Check sheet for the modelled part. Datum: model origin and axes. Units: mm. A direction names the side the tool comes from. Round coordinates to 2 decimals unless told otherwise and drop trailing zeros. Order: outer loops, then holes, each group sorted by start corner. A loop starts at its lowest first (then second) coordinate and runs counter-clockwise, first axis right, second up. Notation, with made-up numbers: (61, -22.75) -> (93, -22.75) arc R14 cw to (93, -7.75) -> close; hole circle Ø1 at (56.25, 59). An arc over 180 degrees is marked (long way). Answer in a Markdown table with one row per item.
from build123d import *

# Parameters (mm, degrees)
BOSS_EXTRUSION_DEPTH     = 5.5
SCHIZZO2_W               = 14.985516936
SCHIZZO2_H               = 7.7
SCHIZZO2_W_2             = 7.7
SCHIZZO2_H_2             = 15.014483064
SCHIZZO2_W_3             = 15.014483064
SCHIZZO2_H_3             = 15
EXTERNAL_EXTRUSION_DEPTH = 13.5
SCHIZZO3_R               = 2.5
CETRAL_HOLE_DEPTH        = 52.71287379
TAGLIO_ESTRUSIONE2_DEPTH = 57.032066134
TAGLIO_ESTRUSIONE3_DEPTH = 57.021948056
TAGLIO_ESTRUSIONE4_DEPTH = 57.021948056
TAGLIO_ESTRUSIONE5_DEPTH = 57.032066134
FORO_PER_VITE_M4_1_D     = 3
FORO_PER_VITE_M4_2_D     = 3
FORO_PER_VITE_M4_3_D     = 3
FORO_PER_VITE_M4_4_D     = 3
RACCORDO1_R              = 4
RACCORDO2_R              = 4
RACCORDO3_R              = 4
RACCORDO4_R              = 4
RACCORDO5_R              = 2
RACCORDO6_R              = 2
RACCORDO7_R              = 2
RACCORDO8_R              = 2
RACCORDO9_R              = 10
RACCORDO17_R             = 10
RACCORDO18_R             = 10
RACCORDO19_R             = 10
RACCORDO20_R             = 10
RACCORDO21_R             = 10
RACCORDO22_DEPTH         = 5.5
RACCORDO23_R             = 10
RACCORDO24_R             = 10
RACCORDO25_R             = 10


with BuildPart() as part:
    # Schizzo1 → Boss extrusion (new body)
    with BuildSketch(Plane(origin=(0, 0, 0), x_dir=(1, 0, 0), z_dir=(0, 1, 0))):
        Polygon((-3.85, -20.28403897), (-3.85, -35.28403897), (3.85, -35.28403897), (3.85, -20.298522034), (15.500302101, -15.451094793), (20.28403897, -3.85), (35.298522034, -3.85), (35.298522034, 3.85), (20.298522034, 3.85), (15.451094793, 15.500302101), (3.85, 20.28403897), (3.85, 35.298522034), (-3.85, 35.298522034), (-3.85, 20.298522034), (-15.500302101, 15.451094793), (-20.28403897, 3.85), (-35.28403897, 3.85), (-35.28403897, -3.85), (-20.298522034, -3.85), (-15.451094793, -15.500302101), align=None)
    extrude(amount=BOSS_EXTRUSION_DEPTH)

    # Schizzo2 → external extrusion (add)
    with BuildSketch(Plane(origin=(0, 5.5, 0), x_dir=(1, 0, 0), z_dir=(0, 1, 0))):
        with Locations((-27.791280502, 0)):
            Rectangle(SCHIZZO2_W, SCHIZZO2_H)
        with Locations((0, 27.791280502)):
            Rectangle(SCHIZZO2_W_2, SCHIZZO2_H_2)
        with Locations((27.791280502, 0)):
            Rectangle(SCHIZZO2_W_3, SCHIZZO2_H)
        with Locations((0, -27.78403897)):
            Rectangle(SCHIZZO2_W_2, SCHIZZO2_H_3)
    extrude(amount=EXTERNAL_EXTRUSION_DEPTH)

    # Schizzo3 → cetral hole (cut, through all)
    with BuildSketch(Plane(origin=(0, 5.5, 0), x_dir=(1, 0, 0), z_dir=(0, 1, 0))):
        with Locations(Location((0, 0, 0), (0, 0, 270))):
            Circle(SCHIZZO3_R)
    extrude(amount=-CETRAL_HOLE_DEPTH, mode=Mode.SUBTRACT)

    # Schizzo4 → Taglio-Estrusione2 (cut, through all)
    with BuildSketch(Plane.XY.offset(3.85)):
        Polygon((35.298522034, 0), (35.298522034, 19), (31.298522034, 0), align=None)
    extrude(amount=-TAGLIO_ESTRUSIONE2_DEPTH, mode=Mode.SUBTRACT)

    # Schizzo5 → Taglio-Estrusione3 (cut, through all)
    with BuildSketch(Plane(origin=(3.85, 0, 0), x_dir=(0, 0, -1), z_dir=(1, 0, 0))):
        Polygon((35.298522034, 0), (35.298522034, 19), (31.298522034, 0), align=None)
    extrude(amount=-TAGLIO_ESTRUSIONE3_DEPTH, mode=Mode.SUBTRACT)

    # Schizzo8 → Taglio-Estrusione4 (cut, through all)
    with BuildSketch(Plane(origin=(0, 0, -3.85), x_dir=(-1, 0, 0), z_dir=(0, 0, -1))):
        Polygon((35.28403897, 0), (35.28403897, 19), (31.28403897, 0), align=None)
    extrude(amount=-TAGLIO_ESTRUSIONE4_DEPTH, mode=Mode.SUBTRACT)

    # Schizzo9 → Taglio-Estrusione5 (cut, through all)
    with BuildSketch(Plane.ZY.offset(3.85)):
        Polygon((35.28403897, 0), (35.28403897, 19), (31.28403897, 0), align=None)
    extrude(amount=-TAGLIO_ESTRUSIONE5_DEPTH, mode=Mode.SUBTRACT)

    # Foro per Vite M4-1 (through all)
    with Locations(Plane.ZY.offset(3.85)):
        with Locations((23.28403897, 15.5), (31.03403897, 15.381977535)):
            Hole(FORO_PER_VITE_M4_1_D / 2)

    # Foro per Vite M4-2 (through all)
    with Locations(Plane.XY.offset(3.85)):
        with Locations((23.28403897, 15.5), (31.03403897, 15.469257355)):
            Hole(FORO_PER_VITE_M4_2_D / 2)

    # Foro per Vite M4-3 (through all)
    with Locations(Plane(origin=(3.85, 0, 0), x_dir=(0, 0, -1), z_dir=(1, 0, 0))):
        with Locations((23.28403897, 15.5), (31.03403897, 15.315212004)):
            Hole(FORO_PER_VITE_M4_3_D / 2)

    # Foro per Vite M4-4 (through all)
    with Locations(Plane(origin=(0, 0, -3.85), x_dir=(-1, 0, 0), z_dir=(0, 0, -1))):
        with Locations((23.298522034, 15.5), (31.048522034, 15.5)):
            Hole(FORO_PER_VITE_M4_4_D / 2)

    # Raccordo1
    raccordo1_edges = [part.edges().sort_by_distance(p)[0] for p in [
        (20.28403897, 19, 0),
    ]]
    fillet(raccordo1_edges, radius=RACCORDO1_R)

    # Raccordo2
    raccordo2_edges = [part.edges().sort_by_distance(p)[0] for p in [
        (0, 19, -20.28403897),
    ]]
    fillet(raccordo2_edges, radius=RACCORDO2_R)

    # Raccordo3
    raccordo3_edges = [part.edges().sort_by_distance(p)[0] for p in [
        (-20.298522034, 19, 0),
    ]]
    fillet(raccordo3_edges, radius=RACCORDO3_R)

    # Raccordo4
    raccordo4_edges = [part.edges().sort_by_distance(p)[0] for p in [
        (0, 19, 20.28403897),
    ]]
    fillet(raccordo4_edges, radius=RACCORDO4_R)

    # Raccordo5
    raccordo5_edges = [part.edges().sort_by_distance(p)[0] for p in [
        (-35.28403897, 19, 0),
    ]]
    fillet(raccordo5_edges, radius=RACCORDO5_R)

    # Raccordo6
    raccordo6_edges = [part.edges().sort_by_distance(p)[0] for p in [
        (0, 19, -35.298522034),
    ]]
    fillet(raccordo6_edges, radius=RACCORDO6_R)

    # Raccordo7
    raccordo7_edges = [part.edges().sort_by_distance(p)[0] for p in [
        (35.298522034, 19, 0),
    ]]
    fillet(raccordo7_edges, radius=RACCORDO7_R)

    # Raccordo8
    raccordo8_edges = [part.edges().sort_by_distance(p)[0] for p in [
        (0, 19, 35.28403897),
    ]]
    fillet(raccordo8_edges, radius=RACCORDO8_R)

    # Raccordo9
    raccordo9_edges = [part.edges().sort_by_distance(p)[0] for p in [
        (3.85, 2.75, 20.298522034),
    ]]
    fillet(raccordo9_edges, radius=RACCORDO9_R)

    # Raccordo17
    raccordo17_edges = [part.edges().sort_by_distance(p)[0] for p in [
        (-3.85, 2.75, 20.28403897),
    ]]
    fillet(raccordo17_edges, radius=RACCORDO17_R)

    # Raccordo18
    raccordo18_edges = [part.edges().sort_by_distance(p)[0] for p in [
        (20.28403897, 2.75, 3.85),
    ]]
    fillet(raccordo18_edges, radius=RACCORDO18_R)

    # Raccordo19
    raccordo19_edges = [part.edges().sort_by_distance(p)[0] for p in [
        (20.298522034, 2.75, -3.85),
    ]]
    fillet(raccordo19_edges, radius=RACCORDO19_R)

    # Raccordo20
    raccordo20_edges = [part.edges().sort_by_distance(p)[0] for p in [
        (3.85, 2.75, -20.28403897),
    ]]
    fillet(raccordo20_edges, radius=RACCORDO20_R)

    # Raccordo21
    raccordo21_edges = [part.edges().sort_by_distance(p)[0] for p in [
        (-3.85, 2.75, -20.298522034),
    ]]
    fillet(raccordo21_edges, radius=RACCORDO21_R)

    # Raccordo22: read off the stored shape, not the designer's step
    # Raccordo22 outline → Raccordo22 (add)
    with BuildSketch(Plane(origin=(0, 0, 0), x_dir=(1, 0, 0), z_dir=(0, 1, 0))):
        with BuildLine():
            add(Edge.make_bspline(
                [(-26.977329566, 3.85), (-20.28403897, 3.85), (-17.732461927, 10.037858563)],
                knots=[0, 0, 0, 1, 1, 1], degree=2, weights=[1, 0.83102772, 1]))
            Line((-26.977329566, 3.85), (-20.28403897, 3.85))
            Line((-20.28403897, 3.85), (-17.732461927, 10.037858563))
        make_face()
    extrude(amount=RACCORDO22_DEPTH)

    # Raccordo23
    raccordo23_edges = [part.edges().sort_by_distance(p)[0] for p in [
        (-20.298522034, 2.75, 3.85),
    ]]
    fillet(raccordo23_edges, radius=RACCORDO23_R)

    # Raccordo24
    raccordo24_edges = [part.edges().sort_by_distance(p)[0] for p in [
        (-15.451094793, 2.75, 15.500302101),
    ]]
    fillet(raccordo24_edges, radius=RACCORDO24_R)

    # Raccordo25
    raccordo25_edges = [part.edges().sort_by_distance(p)[0] for p in [
        (-15.500302101, 2.75, -15.451094793),
        (15.451094793, 2.75, -15.500302101),
        (15.500302101, 2.75, 15.451094793),
    ]]
    fillet(raccordo25_edges, radius=RACCORDO25_R)


solid = part.part
Item 1: Cross-section at A-A (x = 0). Record the boundary of the cut face in (y, z), and give its area (3 significant figures).
Result sheet:
| item | result |
|---|---|
| outline | (0, -31.3) -> (16.59, -34.79) arc R2 ccw to (19, -32.83) -> (19, -24.28) arc R4 ccw to (15, -20.28) -> (5.5, -20.28) -> (5.5, -2.5) -> (0, -2.5) -> close; (0, 2.5) -> (5.5, 2.5) -> (5.5, 20.28) -> (15, 20.28) arc R4 ccw to (19, 24.28) -> (19, 32.82) arc R2 ccw to (16.59, 34.78) -> (0, 31.28) -> close; hole circle Ø3 at (15.32, -31.03); hole circle Ø3 at (15.38, 31.03); hole circle Ø3 at (15.5, -23.28); hole circle Ø3 at (15.5, 23.28) |
| area | 652 mm^2 |
Item 2: Mould release check, pull along Y, two halves, no side actions. Record for faces 6 (the flat face through (0, 19, 28)), 7 (the cylindrical face through (24.783, 15.566, -0.054)), 8 (the flat face through (3.85, 11, -27)): pulls with the +Y half, pulls with the -Y half, needs draft (parallel to the pull), parting line crosses it, or undercut.
Result sheet:
| item | result |
|---|---|
| face 6 | pulls with the +Y half |
| face 7 | undercut |
| face 8 | needs draft |
Item 3: Cross-section at C-C (y = 8.5). Record the boundary of the cut face in (x, z), and give its area (3 significant figures).
Result sheet:
| item | result |
|---|---|
| outline | (-33.07, -3.85) -> (-20.3, -3.85) -> (-20.3, 3.85) -> (-33.07, 3.85) -> close; (-3.85, -33.09) -> (3.85, -33.09) -> (3.85, -20.28) -> (-3.85, -20.28) -> close; (-3.85, 20.28) -> (3.85, 20.28) -> (3.85, 33.07) -> (-3.85, 33.07) -> close; (20.28, -3.85) -> (33.09, -3.85) -> (33.09, 3.85) -> (20.28, 3.85) -> close |
| area | 394 mm^2 |
Item 4: Scan lines: line 1 (Z direction, x = 27.5, y = 3.5); line 2 (Y direction, x = 6.5, z = 14); line 3 (X direction, y = 4.5, z = -26.5). Record each from-to range of solid material in increasing order. Write a range as [from, to].
Result sheet:
| item | result |
|---|---|
| line 1 | z = [-3.85, 3.85] |
| line 2 | y = [0, 5.5] |
| line 3 | x = [-3.86, 3.86] |
Item 5: Cross-section at D-D (z = 5). Record the boundary of the cut face in (x, y), and give its area (3 significant figures).
Result sheet:
| item | result |
|---|---|
| outline | (-22.31, 0) -> (22.32, 0) -> (22.32, 5.5) -> (-22.31, 5.5) -> close |
| area | 245 mm^2 |
Item 6: Cross-section at B-B (y = 12.25). Record the boundary of the cut face in (x, z).
Result sheet:
| item | result |
|---|---|
| outline | (-33.86, -3.85) -> (-20.3, -3.85) -> (-20.3, 3.85) -> (-33.86, 3.85) -> close; (-3.85, -33.88) -> (3.85, -33.88) -> (3.85, -20.28) -> (-3.85, -20.28) -> close; (-3.85, 20.28) -> (3.85, 20.28) -> (3.85, 33.86) -> (-3.85, 33.86) -> close; (20.28, -3.85) -> (33.88, -3.85) -> (33.88, 3.85) -> (20.28, 3.85) -> close |
Item 7: Set-up check for faces 1 (the flat face through (0, 10, -20.284)), 2 (the flat face through (10.831, 2.712, 17.394)), 3 (the flat face through (-3.85, 11, 27)), 4 (the flat face through (-3.85, 11, -28)), 5 (the cylindrical face through (-0.05, 13.85, -31.36)): record each of +Z, -Z, +X, -X, +Y, -Y from which the full face is reachable in a straight line by a thin tool's end or side.
Result sheet:
| item | result |
|---|---|
| face 1 | +X, -X, +Y |
| face 2 | +Z, +X, +Y, -Y |
| face 3 | +Z, -X, +Y |
| face 4 | -Z, -X, +Y |
| face 5 | +X, -X |
Item 8: Depth check by flat-ended pin: P1, Ø4, axis at x = -2, y = 14, coming from the -Z side; P2, Ø2.5, axis at x = -2, y = 10.5, coming from the +Z side; P3, Ø5, axis at y = 15.5, z = -23.28, coming from the +X side; P4, Ø2.5, axis at x = 23.28, y = 15.5, coming from the +Z side. Enter the tip coordinate at first touch or a pass-through.
Result sheet:
| item | result |
|---|---|
| P1 | stops at z = -34.67 |
| P2 | stops at z = 33.76 |
| P3 | stops at x = 3.85 |
| P4 | passes through |
